```python
from build123d import *

# Parameters (mm, degrees)
ESTRUSIONE_ESTRUSIONE1_DEPTH = 14
SVUOTA2_START                = 1.5
SVUOTA2_DEPTH                = 11


# Read off the part's stored shape, not the designer's step: Svuota2
with BuildPart() as part:
    # Schizzo1 → Estrusione-Estrusione1 (new body)
    with BuildSketch(Plane.XY):
        with BuildLine():
            Line((0, 7), (0, 2))
            ThreePointArc((0, 2), (0.585786438, 0.585786438), (2, 0))
            Line((2, 0), (7, 0))
            Line((7, 0), (12, -3.5))
            ThreePointArc((12, -3.5), (14.128037504, -3.705312505), (14.5, -1.6))
            Line((14.5, -1.6), (8.5, 8.4))
            Line((8.5, 8.4), (2, 8.4))
            Line((2, 8.4), (2, 7))
            Line((2, 7), (0, 7))
        make_face()
    extrude(amount=ESTRUSIONE_ESTRUSIONE1_DEPTH)

    # Svuota2 outline → Svuota2 (cut)
    with BuildSketch(Plane.XY.offset(SVUOTA2_START)):
        with BuildLine():
            Line((3.5, 5.5), (0, 5.5))
            Line((0, 5.5), (0, 2))
            ThreePointArc((0, 2), (0.585786438, 0.585786438), (2, 0))
            Line((2, 0), (7, 0))
            Line((7, 0), (12, -3.5))
            ThreePointArc((12, -3.5), (14.128037504, -3.705312505), (14.5, -1.6))
            ThreePointArc((14.5, -1.6), (13.569534227, -0.926722507), (12.429297297, -1.064304775))
            Line((12.429297297, -1.064304775), (7.650714432, 6.9))
            Line((7.650714432, 6.9), (3.5, 6.9))
            Line((3.5, 6.9), (3.5, 5.5))
        make_face()
    extrude(amount=SVUOTA2_DEPTH, mode=Mode.SUBTRACT)


solid = part.part
```
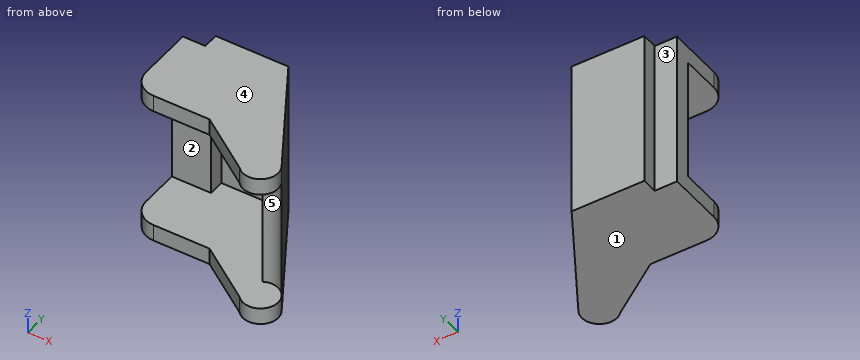
For this review, take the finished solid that the model builds, in its own axes (mm). Face numbers are marked on the shaded views. A direction names the side the tool comes from. Coordinates: 2 decimals unless noted, no trailing zeros. Order: outer loops, then holes, each group sorted by start corner. A loop starts at its lowest first (then second) coordinate and runs counter-clockwise, first axis right, second up. Notation, with made-up numbers: (28, -15.75) - (32, -15.75) arc R12 cw to (32, -10.75) - close; hole circle Ø6 at (-12.75, 47). An arc over 180 degrees is marked (long way). Answer as a JSON object with one key per item and string values. Group by question number.
1. The part is to be moulded in two halves that separate along X. For the marked faces 4 and 5, say which applies: pulls with the +X half, pulls with the -X half, needs draft (parallel to the pull), parting line crosses it, or undercut.
2. We need section B-B on z = 5.75. State the section outline as (x, y) points.
3. We need section D-D on y = 1.5. State the section outline as (x, z) points, then the cut area to 3 significant figures.
4. We need section C-C on x = 5.25. State the section outline as (y, z) points, then the cut area to 3 significant figures.
5. Clearance check with flat-ended pins moving along their axes: P1, Ø1.6, axis at x = 5, z = 0.5, coming from the -Y side; P2, Ø1, axis at x = 1.5, z = 9, coming from the -Y side; P3, Ø0.7, axis at y = 6.5, z = 5.5, coming from the +X side. State where each tip first meets the part, or that it passes through.
6. For the marked faces 1, 2 and 3, list the 3-axis set-ups (+Z, -Z, +X, -X, +Y, -Y) from which the entire face can be reached by the end or side of a thin tool; tool diameter is ignored.
7. We need section A-A on y = -2. State the section outline as (x, z) points, then the cut area to 3 significant figures.
8. For probe 1 along Z at (x, y) = (5, 6.5); probe 2 along Y at (x, z) = (4, 4); probe 3 along Y at (x, z) = (0.5, 4.75), list the stretches that pass through material, from the lowest coordinate up.
Final values:
{
 "1": {"face 4": "needs draft", "face 5": "undercut"},
 "2": {"outline": "(0, 5.5) - (3.5, 5.5) - (3.5, 6.9) - (7.65, 6.9) - (12.43, -1.06) arc R1.57 cw to (14.5, -1.6) - (8.5, 8.4) - (2, 8.4) - (2, 7) - (0, 7) - close"},
 "3": {"outline": "(0.06, 0) - (12.64, 0) - (12.64, 14) - (0.06, 14) - (0.06, 12.5) - (10.89, 12.5) - (10.89, 1.5) - (0.06, 1.5) - close", "area": "57.0 mm²"},
 "4": {"outline": "(0, 0) - (8.4, 0) - (8.4, 14) - (0, 14) - (0, 12.5) - (6.9, 12.5) - (6.9, 1.5) - (0, 1.5) - close", "area": "41.7 mm²"},
 "5": {"P1": "y = 0", "P2": "y = 5.5", "P3": "x = 9.85"},
 "6": {"face 1": "-Z, +X, -X, +Y, -Y", "face 2": "-X, -Y", "face 3": "+Z, -Z, -X, +Y"},
 "7": {"outline": "(9.86, 0) - (14.68, 0) - (14.68, 1.5) - (9.86, 1.5) - close; (9.86, 12.5) - (14.68, 12.5) - (14.68, 14) - (9.86, 14) - close", "area": "14.5 mm²"},
 "8": {"probe 1": "0 to 1.5, 12.5 to 14", "probe 2": "6.9 to 8.4", "probe 3": "5.5 to 7"}
}
